Geometry check sheet. Reference: the model listing, model coordinates, mm. Face numbers are marked on the shaded views. A direction names the side the tool comes from. Give positions to 0.01 mm unless a question says otherwise; leave off trailing zeros. Loops run counter-clockwise (first coordinate to the right, second up) from the corner with the lowest first, then second, coordinate; pieces in that order, holes last. Notation, with made-up numbers: (11, -18) -> (28, -18) arc R23 ccw to (28, -5) -> close; hole circle Ø9 at (-35, -19.5). An arc over 180 degrees is marked (long way). Write each question's results on one line, items separated by ' | '. Start each with the question number.
1) Depth check by flat-ended pin: pin 1 (3 mm diameter, centred on y = -3.5, z = 3, fed in from +X); pin 2 (2 mm diameter, centred on x = 13.5, z = 3, fed in from +Y); pin 3 (3 mm diameter, centred on y = -12.5, z = 1.5, fed in from -X); pin 4 (3 mm diameter, centred on y = 15, z = 3, fed in from -X). Enter the tip coordinate at first touch or a pass-through.
2) Sectioned sample at D-D on y = -13.5. Record the cut outline in (x, z).
3) Scan lines: line 1 (Y direction, x = 13.5, z = -3); line 2 (Y direction, x = -14.5, z = -3); line 3 (X direction, y = 14.5, z = 1.75). Record each from-to range of solid material in increasing order. Write a range as from..to.
4) Draft check along Y on the marked faces 4, 5 and 6. Enter one of: pulls with the +Y half, pulls with the -Y half, needs draft (parallel to the pull), parting line crosses it, or undercut.
5) Sectioned sample at C-C on z = -1.75. Count the separate pieces of the cut face and the enclosed holes in it, then the cut area to 3 significant figures.
6) Set-up check for the marked faces 1, 2 and 3: record each of +Z, -Z, +X, -X, +Y, -Y from which the full face is reachable in a straight line by a thin tool's end or side.
7) Sectioned sample at A-A on y = 0. Record the cut outline in (x, z) (3 decimals).
8) Sectioned sample at B-B on x = 6. Record the cut outline in (y, z).
```python
from build123d import *

# Parameters (mm, degrees)
SKETCH21_W          = 40
SKETCH21_H          = 40
BOSS_EXTRUDE4_DEPTH = 5
FILLET3_R           = 4
SKETCH22_R          = 19.325
CUT_EXTRUDE11_DEPTH = 11
CUT_EXTRUDE12_DEPTH = 7.6
SKETCH30_R          = 1.75
CUT_EXTRUDE13_DEPTH = 10
CIRPATTERN2_COUNT   = 4
BOSS_EXTRUDE3_DEPTH = 2.2
BOSS_EXTRUDE5_REACH = 12


with BuildPart() as part:
    # Sketch21 → Boss-Extrude4 (new body, symmetric)
    with BuildSketch(Plane.XY):
        Rectangle(SKETCH21_W, SKETCH21_H)
    extrude(amount=BOSS_EXTRUDE4_DEPTH, both=True)

    # Fillet3
    fillet3_edges = [part.edges().sort_by_distance(p)[0] for p in [
        (20, -20, 0),
        (-20, -20, 0),
        (-20, 20, 0),
        (20, 20, 0),
    ]]
    fillet(fillet3_edges, radius=FILLET3_R)

    # Sketch22 → Cut-Extrude11 (cut, through all)
    with BuildSketch(Plane.XY.offset(5)):
        Circle(SKETCH22_R)
    extrude(amount=-CUT_EXTRUDE11_DEPTH, mode=Mode.SUBTRACT)

    # Sketch23 → Cut-Extrude12 (cut)
    with BuildSketch(Plane.XY.offset(5)):
        with BuildLine():
            Line((15.262384566, 20), (11.501799696, 16.23941513))
            ThreePointArc((11.501799696, 16.23941513), (0, 19.9), (-11.501799696, 16.23941513))
            Line((-11.501799696, 16.23941513), (-15.262384566, 20))
            Line((-15.262384566, 20), (15.262384566, 20))
        make_face()
    cut_extrude12 = extrude(amount=-CUT_EXTRUDE12_DEPTH, mode=Mode.SUBTRACT)

    # Sketch30 → Cut-Extrude13 (cut)
    with BuildSketch(Plane.XY.offset(5)):
        with Locations((-16, 16)):
            Circle(SKETCH30_R)
    cut_extrude13 = extrude(amount=-CUT_EXTRUDE13_DEPTH, mode=Mode.SUBTRACT)

    # CirPattern2: Cut-Extrude12, Cut-Extrude13 ×4 about axis
    cirpattern2_axis = Axis((0, 0, 0), (0, 0, 1))
    for i in range(1, CIRPATTERN2_COUNT):
        add(cut_extrude12.rotate(cirpattern2_axis, i * 360 / CIRPATTERN2_COUNT), mode=Mode.SUBTRACT)
        add(cut_extrude13.rotate(cirpattern2_axis, i * 360 / CIRPATTERN2_COUNT), mode=Mode.SUBTRACT)

    # Sketch20 → Boss-Extrude3 (add)
    with BuildSketch(Plane(origin=(0, 0, -5), x_dir=(-1, 0, 0), z_dir=(0, 0, -1))):
        with BuildLine():
            Line((6.425058848, 8.928528367), (10.599461946, 16.158806623))
            ThreePointArc((10.599461946, 16.158806623), (9.6625, 16.735940928), (8.694206057, 17.258806623))
            Line((8.694206057, 17.258806623), (4.51980296, 10.028528367))
            ThreePointArc((4.51980296, 10.028528367), (-5.5, 9.526279442), (-10.944861808, 1.1))
            Line((-10.944861808, 1.1), (-19.293668003, 1.1))
            ThreePointArc((-19.293668003, 1.1), (-19.325, 0), (-19.293668003, -1.1))
            Line((-19.293668003, -1.1), (-10.944861808, -1.1))
            ThreePointArc((-10.944861808, -1.1), (-5.5, -9.526279442), (4.51980296, -10.028528367))
            Line((4.51980296, -10.028528367), (8.694206057, -17.258806623))
            ThreePointArc((8.694206057, -17.258806623), (9.6625, -16.735940928), (10.599461946, -16.158806623))
            Line((10.599461946, -16.158806623), (6.425058848, -8.928528367))
            ThreePointArc((6.425058848, -8.928528367), (11, 0), (6.425058848, 8.928528367))
        make_face()
    extrude(amount=-BOSS_EXTRUDE3_DEPTH)

    # Sketch31 → Boss-Extrude5 (add, up to next)
    with BuildSketch(Plane.XY.offset(5), mode=Mode.PRIVATE) as boss_extrude5_sk1:
        with BuildLine():
            Line((-14.240301081, 13.900497298), (-20, 8))
            Line((-20, 8), (-20, -8))
            Line((-20, -8), (-14.240301081, -13.900497298))
            ThreePointArc((-14.240301081, -13.900497298), (-19.9, 0), (-14.240301081, 13.900497298))
        make_face()
    boss_extrude5_tool1 = extrude(boss_extrude5_sk1.sketch, amount=-BOSS_EXTRUDE5_REACH, mode=Mode.PRIVATE) - part.part
    add(boss_extrude5_tool1.solids().sort_by_distance((-19.928391, 0, 5))[0])


solid = part.part
```
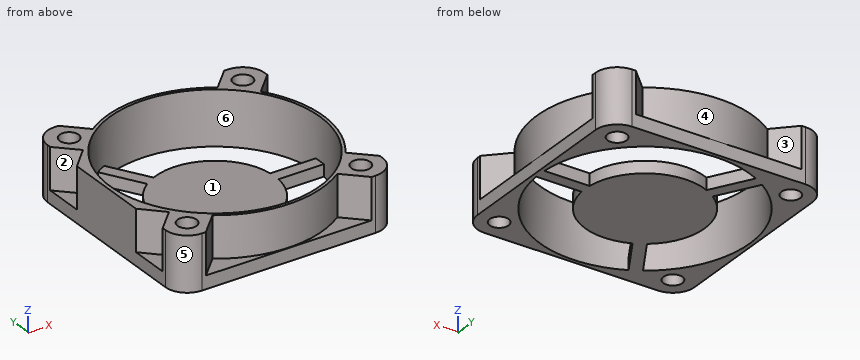
Result:
1) pin 1: x = 19.8 | pin 2: y = 19.24 | pin 3: x = -18.74 | pin 4: x = -20
2) outline: (-20, -5) -> (-13.83, -5) -> (-13.83, 5) -> (-18.24, 5) -> (-18.24, -2.6) -> (-20, -2.6) -> close; (-9.06, -5) -> (-6.52, -5) -> (-6.52, -2.8) -> (-9.06, -2.8) -> close; (13.83, -5) -> (20, -5) -> (20, -2.6) -> (18.24, -2.6) -> (18.24, 5) -> (13.83, 5) -> close
3) line 1: -20..-13.83, -1.1..1.1, 13.83..20 | line 2: -20..-16.9, -15.1..-12.78, 12.78..15.1, 16.9..20 | line 3: -19.24..-16.9, -15.1..-12.78, 12.78..15.1, 16.9..19.24
4) face 4: pulls with the +Y half | face 5: pulls with the -Y half | face 6: undercut
5) separate pieces: 1 | enclosed holes: 5 | area: 218 mm^2
6) face 1: +Z | face 2: +Z, -X | face 3: +Z, +Y
7) outline: (-20, -5) -> (-19.325, -5) -> (-19.325, 5) -> (-20, 5) -> close; (-11, -5) -> (20, -5) -> (20, -2.6) -> (19.9, -2.6) -> (19.9, 5) -> (19.325, 5) -> (19.325, -2.8) -> (-11, -2.8) -> close
8) outline: (-20, -5) -> (-18.37, -5) -> (-18.37, 5) -> (-18.97, 5) -> (-18.97, -2.6) -> (-20, -2.6) -> close; (-9.22, -5) -> (9.22, -5) -> (9.22, -2.8) -> (-9.22, -2.8) -> close; (18.37, -5) -> (20, -5) -> (20, -2.6) -> (18.97, -2.6) -> (18.97, 5) -> (18.37, 5) -> close
